```python
from build123d import *

# Parameters (mm, degrees)
SKETCH_4_W           = 400
SKETCH_4_H           = 300
EXTRUDE_1_DEPTH      = 150
SKETCH_5_R           = 48.25
CUT_EXTRUDE_1_DEPTH  = 42.3
SKETCH_6_W           = 96.5
SKETCH_6_H           = 19.3
CUT_EXTRUDE_2_DEPTH  = 391.512483795
CUT_EXTRUDE_3_DEPTH  = 453.769256907
SKETCH_8_W           = 326
SKETCH_8_H           = 226
CUT_EXTRUDE_5_DEPTH  = 10
SKETCH_9_R           = 48.25
CUT_EXTRUDE_6_DEPTH  = 10
CHAMFER_START        = 259.807621135
CHAMFER_1_OUTLINE_W  = 65
CHAMFER_1_OUTLINE_H  = 74
CHAMFER_1_DEPTH      = 30.192378865
CHAMFER_START_2      = -290
CHAMFER_2_OUTLINE_W  = 64
CHAMFER_2_OUTLINE_H  = 74
CHAMFER_2_DEPTH      = 30.192378865
CHAMFER_3_OUTLINE_W  = 64
CHAMFER_3_OUTLINE_H  = 74
CHAMFER_3_DEPTH      = 30.192378865
CHAMFER_4_OUTLINE_W  = 65
CHAMFER_4_OUTLINE_H  = 74
CHAMFER_4_DEPTH      = 30.192378865
SKETCH_10_W          = 400
SKETCH_10_H          = 50
CUT_EXTRUDE_7_DEPTH  = 391.512483795
SKETCH_11_W          = 340
SKETCH_11_H          = 240
CUT_EXTRUDE_8_DEPTH  = 10
SKETCH_12_W          = 400
SKETCH_12_H          = 30
CUT_EXTRUDE_9_DEPTH  = 391.512483795
SKETCH_13_W          = 41.9021645
SKETCH_13_H          = 193.164300696
SKETCH_13_W_2        = 19.3
SKETCH_13_H_2        = 96.5
CUT_EXTRUDE_10_DEPTH = 453.769256907
SKETCH_14_W          = 261.947815576
SKETCH_14_H          = 41.9021645
SKETCH_14_W_2        = 96.5
SKETCH_14_H_2        = 19.3
CUT_EXTRUDE_11_DEPTH = 391.512483795
SKETCH_16_R          = 65
SKETCH_16_R_2        = 48.25
CUT_EXTRUDE_12_DEPTH = 257.708036866
CHAMFER_5_SIZE       = 10
SKETCH_17_W          = 10
SKETCH_17_H          = 96.5
EXTRUDE_4_DEPTH      = 27.7
SKETCH_19_R          = 1.75
EXTRUDE_6_DEPTH      = 12.5
SKETCH_20_W          = 2
SKETCH_20_H          = 27.7
CUT_EXTRUDE_13_DEPTH = 320.065921872
CHAMFER_6_SIZE       = 8
SKETCH_21_W          = 327.675165592
SKETCH_21_H          = 227.528194438
CUT_EXTRUDE_14_DEPTH = 3


with BuildPart() as part:
    # 草图4 → 凸台-拉伸1 (new body)
    with BuildSketch(Plane.XY):
        Rectangle(SKETCH_4_W, SKETCH_4_H)
    extrude(amount=EXTRUDE_1_DEPTH)

    # 草图5 → 切除-拉伸1 (cut)
    with BuildSketch(Plane.XY.offset(150)):
        Circle(SKETCH_5_R)
    extrude(amount=-CUT_EXTRUDE_1_DEPTH, mode=Mode.SUBTRACT)

    # 草图6 → 切除-拉伸2 (cut, through all)
    with BuildSketch(Plane.XZ.offset(150)):
        with Locations((0, 117.35)):
            Rectangle(SKETCH_6_W, SKETCH_6_H)
    extrude(amount=-CUT_EXTRUDE_2_DEPTH, mode=Mode.SUBTRACT)

    # 草图7 → 切除-拉伸3 (cut, through all)
    with BuildSketch(Plane.ZY.offset(200)):
        Polygon((127, -48.25), (107.7, -48.25), (107.7, 48.25), (127, 48.25), (127, 0), align=None)
    extrude(amount=-CUT_EXTRUDE_3_DEPTH, mode=Mode.SUBTRACT)

    # 草图8 → 切除-拉伸5 (cut)
    with BuildSketch(Plane(origin=(0, 0, 0), x_dir=(-1, 0, 0), z_dir=(0, 0, -1))):
        Rectangle(SKETCH_8_W, SKETCH_8_H)
    extrude(amount=-CUT_EXTRUDE_5_DEPTH, mode=Mode.SUBTRACT)

    # 草图9 → 切除-拉伸6 (cut)
    with BuildSketch(Plane.XY.offset(107.7)):
        Circle(SKETCH_9_R)
    extrude(amount=-CUT_EXTRUDE_6_DEPTH, mode=Mode.SUBTRACT)

    # 倒角1: read off the stored shape, not the designer's step
    # 倒角1 outline → 倒角1 (cut)
    with BuildSketch(Plane(origin=(0, 0, 0), x_dir=(0.8164965809277258, -0.40824829046386313, -0.40824829046386313), z_dir=(0.5773502691896258, 0.5773502691896258, 0.5773502691896258)).offset(CHAMFER_START)):
        with Locations((30.5, 0)):
            Rectangle(CHAMFER_1_OUTLINE_W, CHAMFER_1_OUTLINE_H)
    extrude(amount=CHAMFER_1_DEPTH, mode=Mode.SUBTRACT)

    # 倒角2: read off the stored shape, not the designer's step
    # 倒角2 outline → 倒角2 (cut)
    with BuildSketch(Plane(origin=(0, 0, 0), x_dir=(0.8164965809277258, 0.40824829046386313, 0.40824829046386313), z_dir=(0.5773502691896258, -0.5773502691896258, -0.5773502691896258)).offset(CHAMFER_START_2)):
        with Locations((-31, 0)):
            Rectangle(CHAMFER_2_OUTLINE_W, CHAMFER_2_OUTLINE_H)
    extrude(amount=CHAMFER_2_DEPTH, mode=Mode.SUBTRACT)

    # 倒角3: read off the stored shape, not the designer's step
    # 倒角3 outline → 倒角3 (cut)
    with BuildSketch(Plane(origin=(0, 0, 0), x_dir=(0.8164965809277258, -0.40824829046386313, 0.40824829046386313), z_dir=(0.5773502691896258, 0.5773502691896258, -0.5773502691896258)).offset(CHAMFER_START_2)):
        with Locations((-31, 0)):
            Rectangle(CHAMFER_3_OUTLINE_W, CHAMFER_3_OUTLINE_H)
    extrude(amount=CHAMFER_3_DEPTH, mode=Mode.SUBTRACT)

    # 倒角4: read off the stored shape, not the designer's step
    # 倒角4 outline → 倒角4 (cut)
    with BuildSketch(Plane(origin=(0, 0, 0), x_dir=(0.8164965809277258, 0.40824829046386313, -0.40824829046386313), z_dir=(0.5773502691896258, -0.5773502691896258, 0.5773502691896258)).offset(CHAMFER_START)):
        with Locations((30.5, 0)):
            Rectangle(CHAMFER_4_OUTLINE_W, CHAMFER_4_OUTLINE_H)
    extrude(amount=CHAMFER_4_DEPTH, mode=Mode.SUBTRACT)

    # 草图10 → 切除-拉伸7 (cut, through all)
    with BuildSketch(Plane(origin=(0, 150, 0), x_dir=(1, 0, 0), z_dir=(0, 1, 0))):
        with Locations((0, -25)):
            Rectangle(SKETCH_10_W, SKETCH_10_H)
    extrude(amount=-CUT_EXTRUDE_7_DEPTH, mode=Mode.SUBTRACT)

    # 草图11 → 切除-拉伸8 (cut)
    with BuildSketch(Plane(origin=(0, 0, 50), x_dir=(-1, 0, 0), z_dir=(0, 0, -1))):
        Rectangle(SKETCH_11_W, SKETCH_11_H)
    extrude(amount=-CUT_EXTRUDE_8_DEPTH, mode=Mode.SUBTRACT)

    # 草图12 → 切除-拉伸9 (cut, through all)
    with BuildSketch(Plane(origin=(0, 150, 0), x_dir=(1, 0, 0), z_dir=(0, 1, 0))):
        with Locations((0, -65)):
            Rectangle(SKETCH_12_W, SKETCH_12_H)
    extrude(amount=-CUT_EXTRUDE_9_DEPTH, mode=Mode.SUBTRACT)

    # 草图13 → 切除-拉伸10 (cut, through all)
    with BuildSketch(Plane(origin=(200, 0, 0), x_dir=(0, 0, -1), z_dir=(1, 0, 0))):
        with Locations((-117.35, 0)):
            Rectangle(SKETCH_13_W, SKETCH_13_H)
        with Locations((-117.35, 0)):
            Rectangle(SKETCH_13_W_2, SKETCH_13_H_2, mode=Mode.SUBTRACT)
    extrude(amount=-CUT_EXTRUDE_10_DEPTH, mode=Mode.SUBTRACT)

    # 草图14 → 切除-拉伸11 (cut, through all)
    with BuildSketch(Plane.XZ.offset(150)):
        with Locations((0, 117.35)):
            Rectangle(SKETCH_14_W, SKETCH_14_H)
        with Locations((0, 117.35)):
            Rectangle(SKETCH_14_W_2, SKETCH_14_H_2, mode=Mode.SUBTRACT)
    extrude(amount=-CUT_EXTRUDE_11_DEPTH, mode=Mode.SUBTRACT)

    # 草图16 → 切除-拉伸12 (cut, through all)
    with BuildSketch(Plane(origin=(0, 0, 138.30108225), x_dir=(-1, 0, 0), z_dir=(0, 0, -1))):
        Circle(SKETCH_16_R)
        Circle(SKETCH_16_R_2, mode=Mode.SUBTRACT)
    extrude(amount=-CUT_EXTRUDE_12_DEPTH, mode=Mode.SUBTRACT)

    # 倒角5
    chamfer_5_edges = [part.edges().sort_by_distance(p)[0] for p in [
        (-165.486953894, -96.582150348, 138.30108225),
        (-165.486953894, 96.582150348, 138.30108225),
        (165.486953894, -96.582150348, 138.30108225),
        (165.486953894, 96.582150348, 138.30108225),
        (-130.973907788, 123.291075174, 138.30108225),
        (130.973907788, 123.291075174, 138.30108225),
        (130.973907788, -123.291075174, 138.30108225),
        (-130.973907788, -123.291075174, 138.30108225),
    ]]
    chamfer(chamfer_5_edges, length=CHAMFER_5_SIZE)

    # 草图17 → 凸台-拉伸4 (add)
    with BuildSketch(Plane.XY.offset(96.39891775)):
        with Locations((49.25, 0)):
            Rectangle(SKETCH_17_W, SKETCH_17_H)
        with Locations((-49.25, 0)):
            Rectangle(SKETCH_17_W, SKETCH_17_H)
    extrude(amount=EXTRUDE_4_DEPTH)

    # 草图19 → 凸台-拉伸6 (add)
    with BuildSketch(Plane.XY.offset(96.39891775)):
        with Locations(Location((-15.0260191, -15.0260191, 0), (0, 0, 180))):
            Circle(SKETCH_19_R)
        with Locations(Location((-21.25, 0, 0), (0, 0, 180))):
            Circle(SKETCH_19_R)
        with Locations(Location((-15.0260191, 15.0260191, 0), (0, 0, 180))):
            Circle(SKETCH_19_R)
        with Locations(Location((15.0260191, 15.0260191, 0), (0, 0, 180))):
            Circle(SKETCH_19_R)
        with Locations(Location((21.25, 0, 0), (0, 0, 180))):
            Circle(SKETCH_19_R)
        with Locations(Location((15.0260191, -15.0260191, 0), (0, 0, 180))):
            Circle(SKETCH_19_R)
        with Locations(Location((0, -21.25, 0), (0, 0, 180))):
            Circle(SKETCH_19_R)
        with Locations(Location((0, 21.25, 0), (0, 0, 180))):
            Circle(SKETCH_19_R)
    extrude(amount=EXTRUDE_6_DEPTH)

    # 草图20 → 切除-拉伸13 (cut, through all)
    with BuildSketch(Plane.XZ.offset(48.25)):
        with Locations((-45.25, 110.24891775)):
            Rectangle(SKETCH_20_W, SKETCH_20_H)
        with Locations((45.25, 110.24891775)):
            Rectangle(SKETCH_20_W, SKETCH_20_H)
    extrude(amount=-CUT_EXTRUDE_13_DEPTH, mode=Mode.SUBTRACT)

    # 倒角6
    chamfer_6_edges = [part.edges().sort_by_distance(p)[0] for p in [
        (54.25, 0, 96.39891775),
        (-54.25, 0, 96.39891775),
    ]]
    chamfer(chamfer_6_edges, length=CHAMFER_6_SIZE)

    # 草图21 → 切除-拉伸14 (cut)
    with BuildSketch(Plane(origin=(0, 0, 80), x_dir=(-1, 0, 0), z_dir=(0, 0, -1))):
        Rectangle(SKETCH_21_W, SKETCH_21_H)
    extrude(amount=-CUT_EXTRUDE_14_DEPTH, mode=Mode.SUBTRACT)


solid = part.part
```
Check sheet for the modelled part. Datum: model origin and axes. Units: mm. A direction names the side the tool comes from. Round coordinates to 2 decimals unless told otherwise and drop trailing zeros. Order: outer loops, then holes, each group sorted by start corner. A loop starts at its lowest first (then second) coordinate and runs counter-clockwise, first axis right, second up.
1) Mould release check, pull along X, two halves, no side actions. Record for faces 1 (the flat face through (166, -96.582, 113)), 2 (the flat face through (-181, 134, 135)), 3 (the flat face through (46.25, -1, 110)): +X half, -X half, draft (parallel to the pull), parting line (faces both ways), or undercut.
2) Tool access check on faces 4 (the flat face through (3, -69, 138.301)), 5 (the flat face through (-130.974, 123, 112)), 6 (the flat face through (58.194, -0.675, 100.455)), 7 (the flat face through (-50, 1, 124.099)), 8 (the flat face through (-51, 48.25, 107)). Record the directions out of +Z, -Z, +X, -X, +Y, -Y that give a thin tool (end or side, any length) a straight path to the whole face; none if there is none.
3) Go/stop test with flat-tipped pins: pin 1 Ø2 at (x, y) = (27.5, 25) entering from -Z; pin 2 Ø4 at (x, y) = (-14.5, -16) entering from +Z; pin 3 Ø14 at (y, z) = (-10.5, 109.5) entering from +X. Record where each tip stops, or that it passes through.
4) Scan lines: line 1 (Y direction, x = 0, z = 143); line 2 (Z direction, x = 39, y = -72.5); line 3 (Z direction, x = 180, y = 52). Record each from-to range of solid material in increasing order.
5) Section check B-B (x = 172). Record the boundary of the cut face in (y, z).
6) Section check A-A (z = 116). Record the boundary of the cut face in (x, y).
Result:
1. face 1: draft
1. face 2: -X half
1. face 3: undercut
2. face 4: none
2. face 5: +Y, -Y
2. face 6: +X, +Y, -Y
2. face 7: +X, -X, +Y, -Y
2. face 8: +X, -X, +Y
3. pin 1: stops at z = 83
3. pin 2: stops at z = 108.9
3. pin 3: stops at x = 56.15
4. line 1: y = -150 to -65, 65 to 150
4. line 2: z = 83 to 96.4, 138.3 to 150
4. line 3: z = 80 to 96.4, 138.3 to 150
5. outline: (-150, 80) - (150, 80) - (150, 128) - (128, 150) - (-128, 150) - (-150, 128) - close; hole (-96.58, 96.4) - (96.58, 96.4) - (96.58, 128.3) - (86.58, 138.3) - (-86.58, 138.3) - (-96.58, 128.3) - close
6. outline: (-200, -134) - (-184, -150) - (-130.97, -150) - (-130.97, -96.58) - (-200, -96.58) - close; (-200, 96.58) - (-130.97, 96.58) - (-130.97, 150) - (-184, 150) - (-200, 134) - close; (-54.25, -48.25) - (-46.25, -48.25) - (-46.25, 48.25) - (-54.25, 48.25) - close; (46.25, -48.25) - (54.25, -48.25) - (54.25, 48.25) - (46.25, 48.25) - close; (130.97, -150) - (184, -150) - (200, -134) - (200, -96.58) - (130.97, -96.58) - close; (130.97, 96.58) - (200, 96.58) - (200, 134) - (184, 150) - (130.97, 150) - close
